Read the model definition and answer for the solid it produces. Units are mm, in the model's axes. Face numbers are marked on the shaded views. A direction names the side the tool comes from. Give positions to 0.01 mm unless a question says otherwise; leave off trailing zeros. Order: outer loops, then holes, each group sorted by start corner. A loop starts at its lowest first (then second) coordinate and runs counter-clockwise, first axis right, second up.
Item 1: A cutting plane is placed at B-B (x = -32.5). Write down the section's boundary in (y, z), plus the area to 3 significant figures.
Item 2: A cutting plane is placed at A-A (y = -28). Write down the section's boundary in (x, z), plus the area to 3 significant figures.
Item 3: Given pin 1 Ø13.5 at (y, z) = (-20.5, 23) entering from +X; pin 2 Ø1.5 at (x, y) = (-46.5, -24.5) entering from +Z; pin 3 Ø12 at (y, z) = (-16.5, 14) entering from -X; pin 4 Ø3.5 at (x, y) = (-43.73, -26.54) entering from +Z, each flat-ended and moving along its own axis, determine where each tip first touches the part or whether it passes through.
Item 4: Find the intervals of material crossed by line 1 along Y through (x, z) = (-22.5, 7.5); line 2 along Z through (x, y) = (-55.5, -28.5); line 3 along X through (y, z) = (-19, 19), in increasing order.
Item 5: Which of the six approach directions +Z, -Z, +X, -X, +Y, -Y give full straight-line access (tool end or side, diameter ignored) to the marked faces 1, 2 and 3?
Item 6: A cutting plane is placed at C-C (z = 17). Write down the section's boundary in (x, y), plus the area to 3 significant figures.
Item 7: A cutting plane is placed at D-D (y = -23.5). Write down the section's boundary in (x, z).
from build123d import *

# Parameters (mm, degrees)
F0_W     = 40.386
F0_H     = 12.446
F1_DEPTH = 31.75
F0_W_2   = 50.8
F0_H_2   = 37.592
F2_DEPTH = 6.35
F3_R     = 2.06375
F4_DEPTH = 62.67391


with BuildPart() as f1:
    # F0 (on Front) → F1 (new body)
    with BuildSketch(Plane.XZ):
        with Locations((-43.728333, 25.020055)):
            Rectangle(F0_W, F0_H)
    extrude(amount=F1_DEPTH)

    # F0 (on Front) → F2 (join)
    with BuildSketch(Plane.XZ):
        with Locations((-44.247495, 24.36066)):
            Rectangle(F0_W_2, F0_H_2)
        with Locations((-43.728333, 25.020055)):
            Rectangle(F0_W, F0_H, mode=Mode.SUBTRACT)
    extrude(amount=F2_DEPTH)

    # F3 (on face) → F4 (cut)
    with BuildSketch(Plane(origin=(0, 0, 18.797055), x_dir=(1, 0, 0), z_dir=(0, 0, -1))):
        with Locations((-43.728333, 26.543)):
            Circle(F3_R)
    extrude(amount=-F4_DEPTH, mode=Mode.SUBTRACT)


solid = f1.part
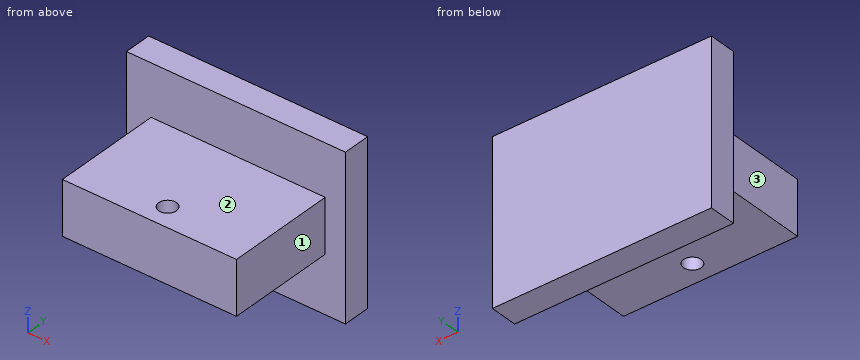
Response values:
1. outline: (-31.75, 18.8) - (-6.35, 18.8) - (-6.35, 5.56) - (0, 5.56) - (0, 43.16) - (-6.35, 43.16) - (-6.35, 31.24) - (-31.75, 31.24) - close
1. area: 555 mm2
2. outline: (-63.92, 18.8) - (-45.19, 18.8) - (-45.19, 31.24) - (-63.92, 31.24) - close; (-42.27, 18.8) - (-23.54, 18.8) - (-23.54, 31.24) - (-42.27, 31.24) - close
2. area: 466 mm2
3. pin 1: stops at x = -23.54
3. pin 2: stops at z = 31.24
3. pin 3: stops at x = -63.92
3. pin 4: passes through
4. line 1: y = -6.35 to 0
4. line 2: z = 18.8 to 31.24
4. line 3: x = -63.92 to -23.54
5. face 1: +Z, -Z, +X, -Y
5. face 2: +Z, +X, -X, -Y
5. face 3: +Z, -Z, -X, -Y
6. outline: (-69.65, -6.35) - (-18.85, -6.35) - (-18.85, 0) - (-69.65, 0) - close
6. area: 323 mm2
7. outline: (-63.92, 18.8) - (-23.54, 18.8) - (-23.54, 31.24) - (-63.92, 31.24) - close
